For this review, use the dimensioned drawing (mm, ordinates from the lowest corner) and the shaded views. A direction names the side the tool comes from. Give positions to 0.01 mm unless a question says otherwise; leave off trailing zeros. Write each loop counter-clockwise with the first axis right and the second up, starting at its lowest first coordinate (ties: lowest second). Pieces come first, ordered by that corner, then holes. Notation, with made-up numbers: (85.25, 53) -> (136.25, 53) arc R31 cw to (136.25, 79) -> close; hole circle Ø3 at (-30, 50.5). An arc over 180 degrees is marked (long way). Return JSON: item names as keys, results as strings.
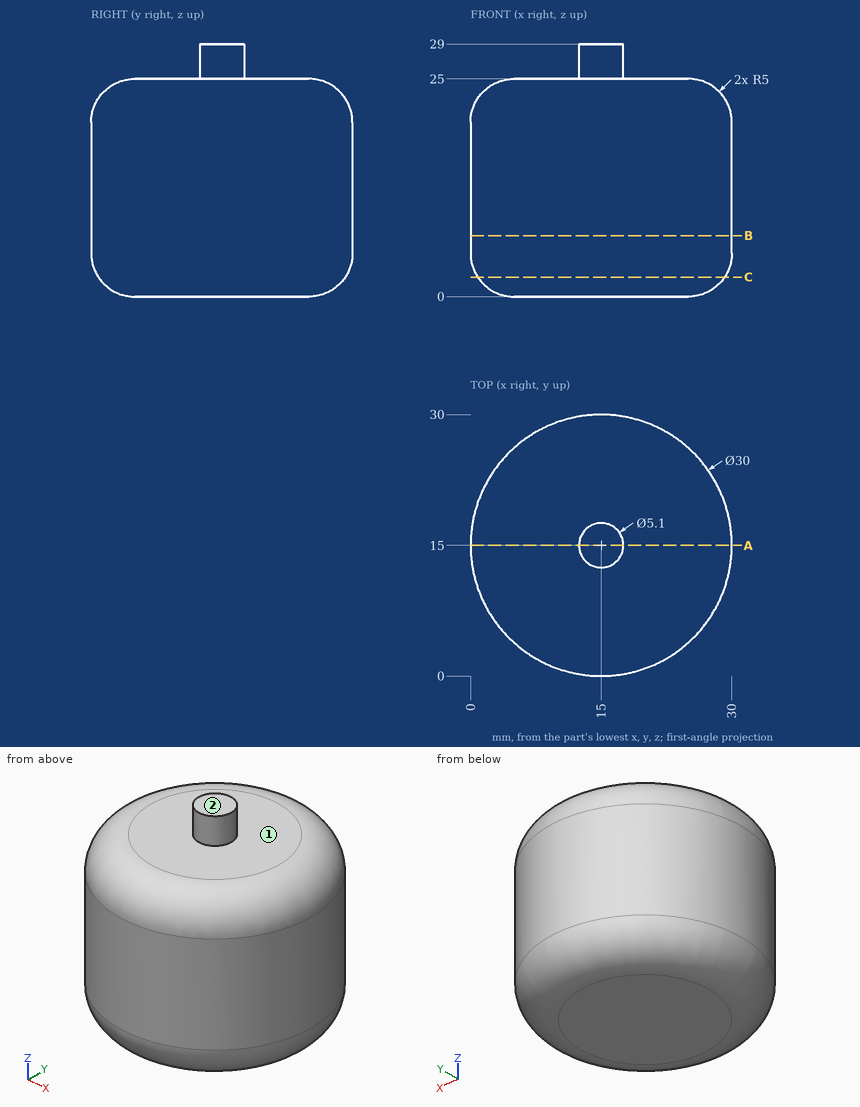
1. Add section C-C, the plane z = 2.25. State the section outline as (x, y) points.
Results found:
{"outline": "circle Ø28.35 at (15, 15)"}
2. Add section B-B, the plane z = 7. State the section outline as (x, y) points.
Results found:
{"outline": "circle Ø30 at (15, 15)"}
3. To check wall thickness, follow probe 1 along X at (y, z) = (14.5, 11.75); probe 2 along Z at (x, y) = (19, 15); probe 3 along Y at (x, z) = (9.5, 23). State the ranges of each line that lie inside material, in increasing order.
Results found:
{"probe 1": "x = 0.01 to 29.99", "probe 2": "z = 0 to 25", "probe 3": "y = 2.13 to 27.87"}
4. For the marked faces 1 and 2, list the 3-axis set-ups (+Z, -Z, +X, -X, +Y, -Y) from which the entire face can be reached by the end or side of a thin tool; tool diameter is ignored.
Results found:
{"face 1": "+Z", "face 2": "+Z, +X, -X, +Y, -Y"}
5. Add section A-A, the plane y = 15. State the section outline as (x, z) points, plus the area to 3 significant figures.
Results found:
{"outline": "(0, 5) arc R5 ccw to (5, 0) -> (25, 0) arc R5 ccw to (30, 5) -> (30, 20) arc R5 ccw to (25, 25) -> (17.55, 25) -> (17.55, 29) -> (12.45, 29) -> (12.45, 25) -> (5, 25) arc R5 ccw to (0, 20) -> close", "area": "749 mm²"}
6. For pin 1 (1.5 mm diameter, centred on y = 16, z = 14.5, fed in from +X); pin 2 (3 mm diameter, centred on x = 6, z = 23.5, fed in from +Y); pin 3 (4 mm diameter, centred on y = 7.5, z = 24.5, fed in from +X), all flat-tipped, find the tip position at first contact; note any pin that passes through.
Results found:
{"pin 1": "stops at x = 30", "pin 2": "stops at y = 26.97", "pin 3": "stops at x = 27.59"}
